from build123d import *

# Parameters (mm, degrees)
F0_R     = 26.9875
F1_DEPTH = 5.08
F2_ANGLE = 90


with BuildPart() as f1:
    # F0 (on Front) → F1 (new body)
    with BuildSketch(Plane.XZ):
        with BuildLine():
            Line((66.675, 36.5125), (-66.675, 36.5125))
            Line((-66.675, 36.5125), (-66.675, -9.55675))
            ThreePointArc((-66.675, -9.55675), (-58.779844, -28.617344), (-39.71925, -36.5125))
            Line((-39.71925, -36.5125), (39.6875, -36.5125))
            ThreePointArc((39.6875, -36.5125), (58.770544, -28.608044), (66.675, -9.525))
            Line((66.675, -9.525), (66.675, 36.5125))
        make_face()
        with Locations((-31.75, 0)):
            Circle(F0_R, mode=Mode.SUBTRACT)
        with Locations((31.75, 0)):
            Circle(F0_R, mode=Mode.SUBTRACT)
    extrude(amount=F1_DEPTH)


with BuildPart() as f1_1:
    # F2: moved
    add(f1.part.rotate(Axis((0, 0, 36.5125), (1, 0, 0)), F2_ANGLE))


with BuildPart() as f1_2:
    # F3: moved
    add(f1_1.part.moved(Location((0, -35.814, -31.496))))


solid = f1_2.part
Check sheet for the modelled part. Datum: model origin and axes. Units: mm. Give positions to 0.01 mm unless a question says otherwise; leave off trailing zeros. Order: outer loops, then holes, each group sorted by start corner. A loop starts at its lowest first (then second) coordinate and runs counter-clockwise, first axis right, second up. Notation, with made-up numbers: (67.25, -29) - (100.25, -29) arc R17 ccw to (100.25, -18) - close; hole circle Ø9 at (25.5, -18.5). An arc over 180 degrees is marked (long way). Answer as CSV lines item,"result".
1. Section check C-C (z = 1.5). State how many separate pieces and enclosed holes the cut face has, then the cut area to 3 significant figures.
Result sheet:
separate pieces,"1"
enclosed holes,"2"
area,"4,850 mm²"
2. Scan lines: probe 1 along Y at (x, z) = (-31.75, 2.95); probe 2 along X at (y, z) = (-6, 1.9) (3 decimals); probe 3 along X at (y, z) = (-2, 4.35) (3 decimals). Record each from-to range of solid material in increasing order. Write a range as from..to.
Result sheet:
probe 1,"-35.81..-26.29, 27.69..37.21"
probe 2,"-66.675..-57.893, -5.607..5.607, 57.893..66.675"
probe 3,"-66.675..-58.602, -4.898..4.898, 58.602..66.675"
3. Section check D-D (x = -41). Record the boundary of the cut face in (y, z).
Result sheet:
outline,"(-35.81, -0.06) - (-24.65, -0.06) - (-24.65, 5.02) - (-35.81, 5.02) - close; (26.05, -0.06) - (37.18, -0.06) - (37.18, 5.02) - (26.05, 5.02) - close"
4. Section check A-A (x = 31.75). Record the boundary of the cut face in (y, z), then the cut area to 3 significant figures.
Result sheet:
outline,"(-35.81, -0.06) - (-26.29, -0.06) - (-26.29, 5.02) - (-35.81, 5.02) - close; (27.69, -0.06) - (37.21, -0.06) - (37.21, 5.02) - (27.69, 5.02) - close"
area,"96.8 mm²"
5. Go/stop test with a flat-tipped pin: P1, Ø3, axis at y = 20, z = 2, coming from the +X side. Record where the tip stops, or that it passes through.
Result sheet:
P1,"x = 65.37"
6. Section check B-B (y = -13.5). Record the boundary of the cut face in (x, z) (1 decimal), then the cut area to 3 significant figures.
Result sheet:
outline,"(-66.7, -0.1) - (-54.7, -0.1) - (-54.7, 5) - (-66.7, 5) - close; (-8.8, -0.1) - (8.8, -0.1) - (8.8, 5) - (-8.8, 5) - close; (54.7, -0.1) - (66.7, -0.1) - (66.7, 5) - (54.7, 5) - close"
area,"211 mm²"
7. Mould release check, pull along X, two halves, no side actions. Record for faces 1 (the face through (58.56, 29.515, 2.512)), 2 (the face through (56.68, 11.03, 2.51)), 3 (the face through (-66.675, -13, 3)): released by +X, released by -X, zero draft, split by the parting line, or undercut.
Result sheet:
face 1,"released by +X"
face 2,"undercut"
face 3,"released by -X"
